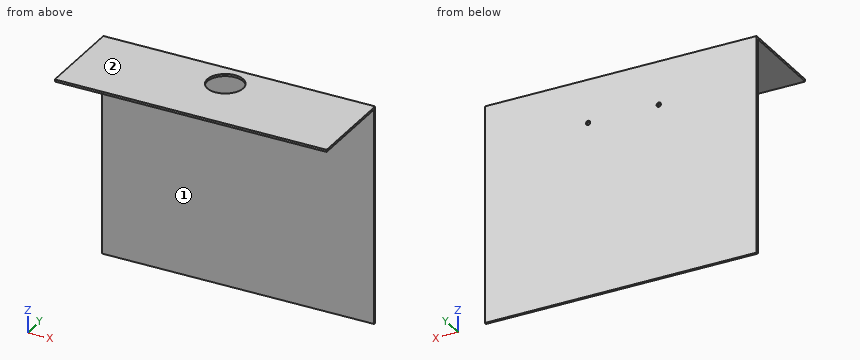
```python
from build123d import *

# Parameters (mm, degrees)
SKETCH1_W           = 250
SKETCH1_H           = 200
BOSS_EXTRUDE1_DEPTH = 2
SKETCH2_W           = 250
SKETCH2_H           = 2
BOSS_EXTRUDE2_DEPTH = 81
SKETCH3_R           = 2
CUT_EXTRUDE1_DEPTH  = 331.740079216
CUT_EXTRUDE2_REACH  = 332.244
SKETCH4_R           = 16.5


with BuildPart() as part:
    # Sketch1 → Boss-Extrude1 (new body)
    with BuildSketch(Plane(origin=(0, 0, 0), x_dir=(1, 0, 0), z_dir=(0, 1, 0))):
        with Locations((125, 100)):
            Rectangle(SKETCH1_W, SKETCH1_H)
    extrude(amount=BOSS_EXTRUDE1_DEPTH)

    # Sketch2 → Boss-Extrude2 (add)
    with BuildSketch(Plane.XZ):
        with Locations((125, -1)):
            Rectangle(SKETCH2_W, SKETCH2_H)
    extrude(amount=BOSS_EXTRUDE2_DEPTH)

    # Sketch3 → Cut-Extrude1 (cut, through all)
    with BuildSketch(Plane(origin=(0, 2, 0), x_dir=(1, 0, 0), z_dir=(0, 1, 0))):
        with Locations(Location((155, 40, 0), (0, 0, 270))):
            Circle(SKETCH3_R)
        with Locations(Location((90, 40, 0), (0, 0, 270))):
            Circle(SKETCH3_R)
    extrude(amount=-CUT_EXTRUDE1_DEPTH, mode=Mode.SUBTRACT)

    # Sketch4 → Cut-Extrude2 (cut, up to next)
    with BuildSketch(Plane.XY, mode=Mode.PRIVATE) as cut_extrude2_sk1:
        with Locations((125, -22)):
            Circle(SKETCH4_R)
    cut_extrude2_tool1 = extrude(cut_extrude2_sk1.sketch, amount=-CUT_EXTRUDE2_REACH, mode=Mode.PRIVATE) & part.part
    add(cut_extrude2_tool1.solids().sort_by_distance((125, -22, 0))[0], mode=Mode.SUBTRACT)


solid = part.part
```
The listing builds one solid part. Answer for the finished solid, in the listing's coordinates (mm). Face numbers are marked on the shaded views. A direction names the side the tool comes from. Coordinates: 2 decimals unless noted, no trailing zeros. Write each loop counter-clockwise with the first axis right and the second up, starting at its lowest first coordinate (ties: lowest second). Pieces come first, ordered by that corner, then holes.
Q1. Which of the six approach directions +Z, -Z, +X, -X, +Y, -Y give full straight-line access (tool end or side, diameter ignored) to the marked faces 1 and 2?
Returned:
face 1: -Z, +X, -X, -Y
face 2: +Z, +X, -X, +Y, -Y
Q2. Find the intervals of material crossed by line 1 along X through (y, z) = (1, -40); line 2 along Z through (x, y) = (155, 0.9); line 3 along Y through (x, z) = (125, -0.7), in increasing order.
Returned:
line 1: x = 0 to 88, 92 to 153, 157 to 250
line 2: z = -200 to -42, -38 to 0
line 3: y = -81 to -38.5, -5.5 to 2
Q3. Section C-C, the plane x = 42.5 is taken. Write down the section's boundary in (y, z), then the cut area to 3 significant figures.
Returned:
outline: (-81, -2) - (0, -2) - (0, -200) - (2, -200) - (2, 0) - (-81, 0) - close
area: 562 mm2
Q4. Section A-A, the plane x = 125 is taken. Write down the section's boundary in (y, z).
Returned:
outline: (-81, -2) - (-38.5, -2) - (-38.5, 0) - (-81, 0) - close; (-5.5, -2) - (0, -2) - (0, -200) - (2, -200) - (2, 0) - (-5.5, 0) - close
Q5. Given P1, Ø4.5, axis at x = 90, z = -40, coming from the -Y side; P2, Ø2, axis at x = 164.5, y = -61, coming from the +Z side; P3, Ø24.5, axis at x = 87.5, y = -51, coming from the -Z side, each flat-ended and moving along its own axis, determine where each tip first touches the part or whether it passes through.
Returned:
P1: stops at y = 0
P2: stops at z = 0
P3: stops at z = -2
Q6. Section B-B, the plane y = -27 is taken. Write down the section's boundary in (x, z).
Returned:
outline: (0, -2) - (109.28, -2) - (109.28, 0) - (0, 0) - close; (140.72, -2) - (250, -2) - (250, 0) - (140.72, 0) - close
Q7. Section D-D, the plane z = -146 is taken. Write down the section's boundary in (x, y), then the cut area to 3 significant figures.
Returned:
outline: (0, 0) - (250, 0) - (250, 2) - (0, 2) - close
area: 500 mm2
